```python
from build123d import *

# Parameters (mm, degrees)
F0_W      = 40
F0_H      = 25
F1_DEPTH  = 6
F2_W      = 6
F2_H      = 25
F3_DEPTH  = 9
F5_DEPTH  = 6
F6_R      = 2.5
F7_DEPTH  = 5
F8_R      = 2.5
F9_DEPTH  = 5
F10_R     = 3
F11_DEPTH = 6.001


with BuildPart() as f1:
    # F0 (on Top) → F1 (new body)
    with BuildSketch(Plane.XY):
        with Locations((-12.984823, 9.274423)):
            Rectangle(F0_W, F0_H)
    extrude(amount=F1_DEPTH)

    # F2 (on face) → F3 (join)
    with BuildSketch(Plane.XY.offset(6)):
        with Locations((4.015177, 9.274423)):
            Rectangle(F2_W, F2_H)
    extrude(amount=F3_DEPTH)

    # F4 (on face) → F5 (join)
    with BuildSketch(Plane.YZ.offset(7.015177)):
        with BuildLine():
            Line((12.774423, 31), (12.774423, 21))
            ThreePointArc((12.774423, 21), (9.274423, 17.5), (5.774423, 21))
            Line((5.774423, 21), (5.774423, 31))
            Line((5.774423, 31), (1.774423, 31))
            Line((1.774423, 31), (-3.225577, 15))
            Line((-3.225577, 15), (21.774423, 15))
            Line((21.774423, 15), (16.774423, 31))
            Line((16.774423, 31), (12.774423, 31))
        make_face()
    extrude(amount=-F5_DEPTH)

    # F6 (on face) → F7 (join)
    with BuildSketch(Plane.XZ.offset(3.225577)):
        with BuildLine():
            Line((7.015177, 15), (7.015177, 0))
            Line((7.015177, 0), (14.015177, 0))
            ThreePointArc((14.015177, 0), (19.920596, 4.938852), (16.104019, 11.624655))
            Line((16.104019, 11.624655), (7.015177, 15))
        make_face()
        with Locations((14.015177, 6)):
            Circle(F6_R, mode=Mode.SUBTRACT)
    extrude(amount=-F7_DEPTH)

    # F8 (on face) → F9 (join)
    with BuildSketch(Plane(origin=(0, 21.774423, 0), x_dir=(-1, 0, 0), z_dir=(0, 1, 0))):
        with BuildLine():
            Line((-7.015177, 0), (-7.015177, 15))
            Line((-7.015177, 15), (-16.104019, 11.624655))
            ThreePointArc((-16.104019, 11.624655), (-19.920596, 4.938852), (-14.015177, 0))
            Line((-14.015177, 0), (-7.015177, 0))
        make_face()
        with Locations((-14.015177, 6)):
            Circle(F8_R, mode=Mode.SUBTRACT)
    extrude(amount=-F9_DEPTH)

    # F10 (on face) → F11 (cut, through all)
    with BuildSketch(Plane.XY.offset(6)):
        with Locations((-7.984823, 9.274423)):
            Circle(F10_R)
        with Locations((-25.484823, 9.274423)):
            Circle(F10_R)
    extrude(amount=-F11_DEPTH, mode=Mode.SUBTRACT)


solid = f1.part
```
The listing builds one solid part. Answer for the finished solid, in the listing's coordinates (mm). A direction names the side the tool comes from. Coordinates: 2 decimals unless noted, no trailing zeros. Loops run counter-clockwise (first coordinate to the right, second up) from the corner with the lowest first, then second, coordinate; pieces in that order, holes last. Notation, with made-up numbers: (75.5, 87) -> (86.5, 87) arc R33 ccw to (86.5, 125) -> close; hole circle Ø6 at (-21.75, 39.25). An arc over 180 degrees is marked (long way). Return JSON: item names as keys, results as strings. Group by question number.
(1) Find the intervals of material crossed by probe 1 along Z at (x, y) = (15, -0.5); probe 2 along X at (y, z) = (2.5, 11); probe 3 along Y at (x, z) = (3.5, 28), in increasing order. Write a range as from..to.
(2) A cutting plane is placed at B-B on z = 19.5. Write down the section's boundary in (x, y).
(3) Given pin 1 Ø5 at (y, z) = (9, 14.5) entering from +X; pin 2 Ø7.5 at (y, z) = (11.5, 20.5) entering from -X; pin 3 Ø7 at (x, y) = (-25.48, 9.27) entering from +Z; pin 4 Ø5.5 at (x, y) = (-7.98, 9.27) entering from +Z, each flat-ended and moving along its own axis, determine where each tip first touches the part or whether it passes through.
(4) A cutting plane is placed at C-C on x = 5. Write down the section's boundary in (y, z), and give its area (3 significant figures).
(5) Determine the mould class of faces 1 (the cylindrical face through (15.86, 19.31, 7.69)), 2 (the cylindrical face through (-27.7, 11.3, 3)), 3 (the flat face through (-9.2, 12.2, 0)) for opening direction Z: released by +Z, released by -Z, zero draft, split by the parting line, or undercut.
(6) Which of the six approach directions +Z, -Z, +X, -X, +Y, -Y give full straight-line access (tool end or side, diameter ignored) to faces 4 (the flat face through (12, 1.774, 8)), 5 (the flat face through (1.015, 9, 16)), 6 (the flat face through (4, 12.774, 26))?
(7) A cutting plane is placed at D-D on y = 1. Write down the section's boundary in (x, z).
(8) A cutting plane is placed at A-A on y = 8.5. Write down the section's boundary in (x, z).
The answers:
{
 "1": {"probe 1": "z = 0.08..3.7, 8.3..12.03", "probe 2": "x = 1.02..7.02", "probe 3": "y = 0.84..5.77, 12.77..17.71"},
 "2": {"outline": "(1.02, -1.82) -> (7.02, -1.82) -> (7.02, 6.11) -> (1.02, 6.11) -> close; (1.02, 12.44) -> (7.02, 12.44) -> (7.02, 20.37) -> (1.02, 20.37) -> close"},
 "3": {"pin 1": "stops at x = 7.02", "pin 2": "stops at x = 1.02", "pin 3": "stops at z = 6", "pin 4": "passes through"},
 "4": {"outline": "(-3.23, 0) -> (21.77, 0) -> (21.77, 15) -> (16.77, 31) -> (12.77, 31) -> (12.77, 21) arc R3.5 cw to (5.77, 21) -> (5.77, 31) -> (1.77, 31) -> (-3.23, 15) -> close", "area": "606 mm^2"},
 "5": {"face 1": "undercut", "face 2": "zero draft", "face 3": "released by -Z"},
 "6": {"face 4": "+Z, -Z, +X", "face 5": "+Z, -X, +Y, -Y", "face 6": "+Z, +X, -X"},
 "7": {"outline": "(-32.98, 0) -> (14.02, 0) arc R6 ccw to (16.1, 11.62) -> (7.02, 15) -> (7.02, 28.52) -> (1.02, 28.52) -> (1.02, 6) -> (-32.98, 6) -> close; hole circle Ø5 at (14.02, 6)"},
 "8": {"outline": "(-32.98, 0) -> (-28.38, 0) -> (-28.38, 6) -> (-32.98, 6) -> close; (-22.59, 0) -> (-10.88, 0) -> (-10.88, 6) -> (-22.59, 6) -> close; (-5.09, 0) -> (7.02, 0) -> (7.02, 17.59) -> (1.02, 17.59) -> (1.02, 6) -> (-5.09, 6) -> close"}
}
